```python
from build123d import *

# Parameters (mm, degrees)
F2_SIZE = 3
F3_R    = 4.99999


# Not quite as in the source:
# - a fillet or chamfer is up to 0.001 mm smaller than in the source, because OpenCascade refuses the exact size


with BuildPart() as f1:
    # F0 (on Front) → F1 (revolve)
    with BuildSketch(Plane.XZ):
        Polygon((-64, 22.25), (-94, 22.25), (-94, 27.25), (-99, 27.25), (-99, 0), (-64, 0), align=None)
    revolve(axis=Axis((-47, 0, 0), (-1, 0, 0)))

    # F2
    f2_edges = [f1.edges().sort_by_distance(p)[0] for p in [
        (-64, 0, -22.25),
    ]]
    chamfer(f2_edges, length=F2_SIZE)

    # F3 (radius 5 in the source; OpenCascade refuses exactly that, so slightly less here)
    f3_edges = [f1.edges().sort_by_distance(p)[0] for p in [
        (-94, 0, -22.25),
    ]]
    fillet(f3_edges, radius=F3_R)


solid = f1.part
```
Design review of the part built by this model. Coordinates are the model's own, in mm. A direction names the side the tool comes from. Coordinates: 2 decimals unless noted, no trailing zeros. Order: outer loops, then holes, each group sorted by start corner. A loop starts at its lowest first (then second) coordinate and runs counter-clockwise, first axis right, second up.
1) Clearance check with flat-ended pins moving along their axes: pin 1 (2 mm diameter, centred on x = -68, y = 18, fed in from +Z); pin 2 (4 mm diameter, centred on x = -84, z = 0, fed in from -Y); pin 3 (5 mm diameter, centred on y = -14.5, z = 13.5, fed in from +X); pin 4 (1 mm diameter, centred on x = -86, y = 9.5, fed in from -Z). State where each tip first meets the part, or that it passes through.
2) Wall thickness on line 1 along Y through (x, z) = (-84, -0.5); line 2 along Y through (x, z) = (-88.5, -12): over which ranges is each line inside the solid? List them lowest first.
3) For faces 1 (the flat face through (-99, 0, 0)), 2 (the cylindrical face through (-78.154, 15.038, -16.399)), list the 3-axis set-ups (+Z, -Z, +X, -X, +Y, -Y) from which the entire face can be reached by the end or side of a thin tool; tool diameter is ignored.
4) Take a section at C-C, the plane x = -74.5. Give the boundary of the cut face in (y, z).
Returned:
1. pin 1: stops at z = 14.35
1. pin 2: stops at y = -22.25
1. pin 3: stops at x = -64
1. pin 4: stops at z = -20.35
2. line 1: y = -22.24 to 22.24
2. line 2: y = -18.74 to 18.74
3. face 1: +Z, -Z, -X, +Y, -Y
3. face 2: +X
4. outline: circle Ø44.5 at (0, 0)
